Can you work these out from the model? Positions are in its coordinate system, mm. Face numbers are marked on the shaded views. A direction names the side the tool comes from. Give positions to 0.01 mm unless a question says otherwise; leave off trailing zeros. Order: outer loops, then holes, each group sorted by start corner. A loop starts at its lowest first (then second) coordinate and runs counter-clockwise, first axis right, second up. Notation, with made-up numbers: M 83,14.25 L 130,14.25 A28 cw 130,48.25 Z; hole C 86.5,10 d8. An arc over 180 degrees is marked long. Use one line per item in the form item = value. Start each with the question number.
1. I want a section at D-D, the plane y = 26. List the corners of the cut face in (x, z) for me, and give its area (3 significant figures).
2. I want a section at C-C, the plane x = 22.5. List the corners of the cut face in (y, z) for me.
3. I need wall thicknesses on L1, parallel to Z at x = 0, y = 2; L2, parallel to Z at x = 0, y = 31.15; L3, parallel to Z at x = -22.5, y = 3.5. Which ranges of each line are inside material? Lowest first, please.
4. I want a section at B-B, the plane z = 12.5. List the corners of the cut face in (x, y) for me.
5. I want a section at A-A, the plane z = 0. List the corners of the cut face in (x, y) for me.
6. For the marked faces 1, 2 and 3, which set-ups out of +Z, -Z, +X, -X, +Y, -Y let a thin tool reach every point of the face, with its end or its side?
7. Will these pins go through, and if not, where does the flat tip stop? P1, Ø4, axis at x = 0, z = -22.5, coming from the +Y side; P2, Ø12, axis at x = 0, y = 25.5, coming from the +Z side; P3, Ø4, axis at x = 1, y = 17, coming from the -Z side.
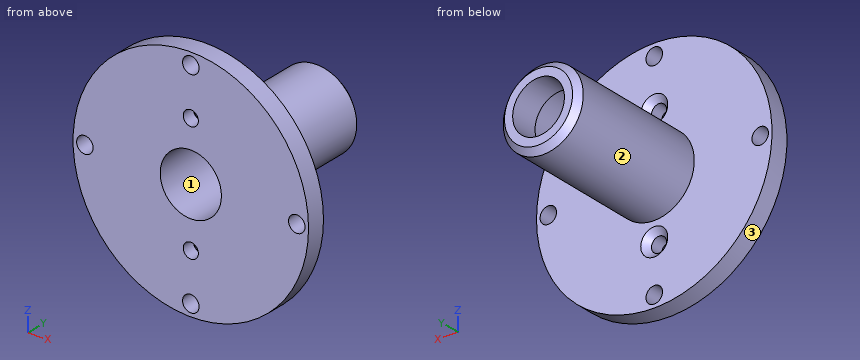
Autodesk Inventor part; units mm, degrees
ref_plane "YZ Plane" through (0, 0, 0) normal (1, 0, 0) x (0, 1, 0)
ref_plane "XZ Plane" through (0, 0, 0) normal (0, 1, 0) x (-1, 0, 0)
ref_plane "XY Plane" through (0, 0, 0) normal (0, 0, 1) x (1, 0, 0)
sketch "Sketch1" plane through (0, 0, 0) normal (0, 0, 1) x (1, 0, 0)
  line L0 (0, 0) -> (25, 0)
  line L1 (25, 0) -> (25, 4)
  line L2 (25, 4) -> (8.5, 4)
  line L3 (8.5, 4) -> (8.5, 35)
  line L4 (8.5, 35) -> (0, 35)
  line L5 (0, 0) -> (6.5, 0)
  line L6 (6.5, 0) -> (6.5, 29)
  line L7 (6.5, 29) -> (5.5, 29)
  line L8 (5.5, 29) -> (5.5, 35)
  line L9 (0, 35) -> (0, 0)
  dimension "d0" = 25
  dimension "d1" = 4
  dimension "d2" = 8.5
  dimension "d3" = 31
  dimension "d4" = 6.5
  dimension "d5" = 29
  dimension "d6" = 5.5
revolve "Revolution1" add sketch "Sketch1" angle 360 about axis through (0, 35, 0) along (0, -1, 0) contours L6 L7 L8 L4 L3 L2 L1 L0
sketch "Sketch2" plane through (0, 4, 0) normal (0, 1, 0) x (1, 0, 0)
  circle A0 centre (0, -22.5) radius 1.75
  circle A1 centre (22.5, 0) radius 1.75
  circle A2 centre (0, 22.5) radius 1.75
  circle A3 centre (-22.5, 0) radius 1.75
  circle A4 centre (0, -12.5) radius 1.6
  circle A5 centre (0, 12.5) radius 1.6
  point P0 (0, 0)
  dimension "d8" = 3.5
  dimension "d9" = 22.5
  dimension "d12" = 360
  dimension "d14" = 3.2
  dimension "d15" = 12.5
  dimension "d18" = 360
extrude "Extrusion1" cut sketch "Sketch2" against normal blind 25.4
chamfer "Chamfer1" distance 1.27 angle 45 2 edges at (-1.6, 4, 12.5) (-1.6, 4, -12.5)
chamfer "Chamfer2" distance 1.27 angle 45 1 edges at (-8.5, 35, 0)
properties part number "MotorMount"
Check result:
q1.outline = C 0,0 d17; hole C 0,0 d13
q1.area = 94.2 mm2
q2.outline = M 0,-10.9 L 4,-10.9 L 4,-1.75 L 0,-1.75 Z; M 0,1.75 L 4,1.75 L 4,10.9 L 0,10.9 Z
q3.L1 = -25 to -24.25, -20.75 to -14.1, -10.9 to -6.5, 6.5 to 10.9, 14.1 to 20.75, 24.25 to 25
q3.L2 = -8.5 to -5.5, 5.5 to 8.5
q3.L3 = -10.9 to -1.75, 1.75 to 10.9
q4.outline = M -21.65,0 L -1.6,0 L -1.6,2.73 L -2.87,4 L -21.65,4 Z; M 1.6,0 L 21.65,0 L 21.65,4 L 2.87,4 L 1.6,2.73 Z
q5.outline = M -25,0 L -24.25,0 L -24.25,4 L -25,4 Z; M -20.75,0 L -6.5,0 L -6.5,29 L -5.5,29 L -5.5,35 L -7.23,35 L -8.5,33.73 L -8.5,4 L -20.75,4 Z; M 5.5,29 L 6.5,29 L 6.5,0 L 20.75,0 L 20.75,4 L 8.5,4 L 8.5,33.73 L 7.23,35 L 5.5,35 Z; M 24.25,0 L 25,0 L 25,4 L 24.25,4 Z
q6.face_1 = -Y
q6.face_2 = +Y
q6.face_3 = +Y, -Y
q7.P1 = 4
q7.P2 = 8.5
q7.P3 = -8.5
